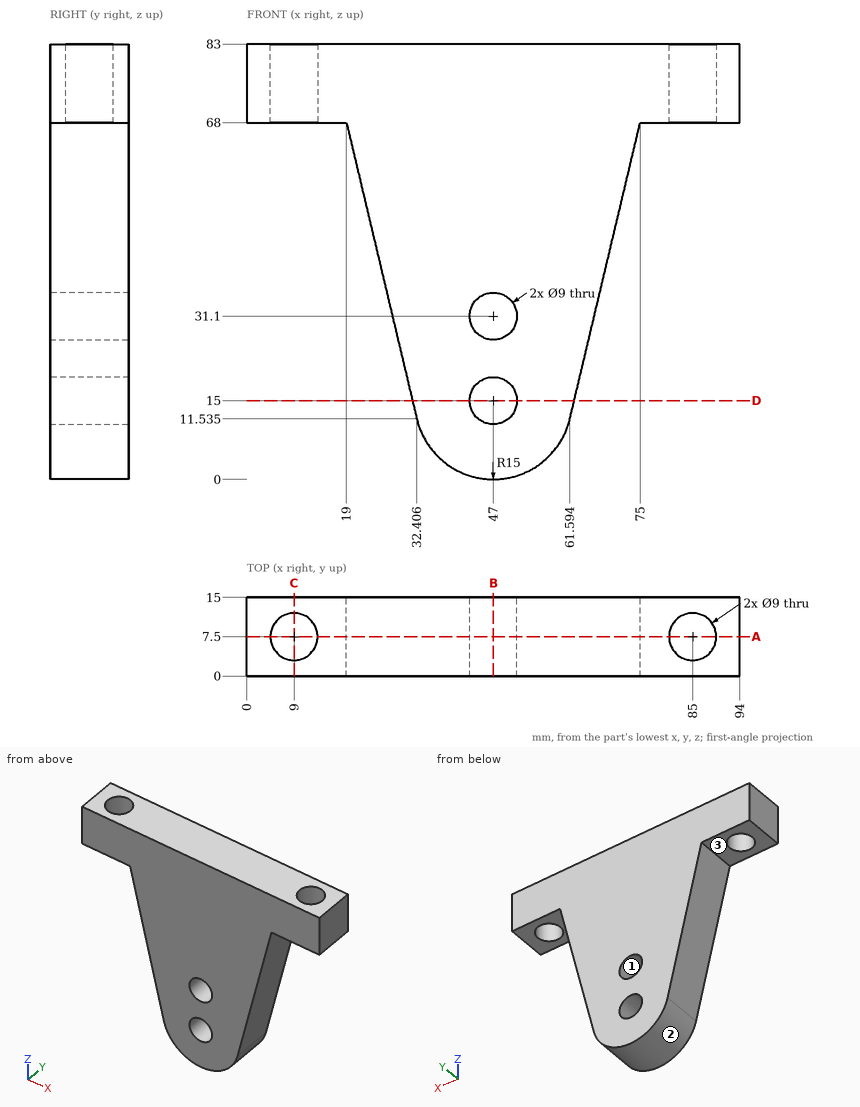
Input: dimensioned drawing with shaded views. Units: mm. Origin: part minimum x, y, z. Coordinates: 2 decimals unless noted, no trailing zeros. Loops run counter-clockwise (first coordinate to the right, second up) from the corner with the lowest first, then second, coordinate; pieces in that order, holes last. Notation, with made-up numbers: M -5,7 L 24,7 A26 ccw 24,25 Z; hole C 2,78.25 d5. An arc over 180 degrees is marked long. Use a Markdown table: item, result. Add a question column.
Q1. Section query A-A, the plane y = 7.5. Return loops of the section in (x, z) (1 decimal).
Q2. Material intervals for L1, parallel to Y at x = 85, z = 79; L2, parallel to Z at x = 50, y = 1 (1 decimal); L3, parallel to X at y = 5.75, z = 15, sorted ascending.
Q3. First-contact query: pin 1 (2 mm diameter, centred on y = 11, z = 55.5, fed in from +X); pin 2 (4.5 mm diameter, centred on x = 81, y = 10, fed in from -Z); pin 3 (3 mm diameter, centred on y = 8.5, z = 48, fed in from -X). Flat tips, straight axial feed; report the tip coordinate or a pass-through.
Q4. Section query B-B, the plane x = 47. Return loops of the section in (y, z).
Q5. Draft query along X for the marked faces 1, 2 and 3. Return one class per face: pulls with the +X half, pulls with the -X half, needs draft (parallel to the pull), parting line crosses it, or undercut.
Q6. Section query C-C, the plane x = 9. Return loops of the section in (y, z).
Q7. Section query D-D, the plane z = 15. Return loops of the section in (x, y).
Result:
| question | item | result |
|---|---|---|
| 1 | outline | M 0,68 L 4.5,68 L 4.5,83 L 0,83 Z; M 13.5,68 L 19,68 L 32.4,11.5 A15 ccw 61.6,11.5 L 75,68 L 80.5,68 L 80.5,83 L 13.5,83 Z; M 89.5,68 L 94,68 L 94,83 L 89.5,83 Z; hole C 47,15 d9; hole C 47,31.1 d9 |
| 2 | L1 | y = 0 to 3, 12 to 15 |
| 2 | L2 | z = 0.3 to 11.6, 18.4 to 27.7, 34.5 to 83 |
| 2 | L3 | x = 31.58 to 42.5, 51.5 to 62.42 |
| 3 | pin 1 | stops at x = 72.27 |
| 3 | pin 2 | stops at z = 68 |
| 3 | pin 3 | stops at x = 23.39 |
| 4 | outline | M 0,0 L 15,0 L 15,10.5 L 0,10.5 Z; M 0,19.5 L 15,19.5 L 15,26.6 L 0,26.6 Z; M 0,35.6 L 15,35.6 L 15,83 L 0,83 Z |
| 5 | face 1 | undercut |
| 5 | face 2 | parting line crosses it |
| 5 | face 3 | needs draft |
| 6 | outline | M 0,68 L 3,68 L 3,83 L 0,83 Z; M 12,68 L 15,68 L 15,83 L 12,83 Z |
| 7 | outline | M 31.58,0 L 42.5,0 L 42.5,15 L 31.58,15 Z; M 51.5,0 L 62.42,0 L 62.42,15 L 51.5,15 Z |
